from build123d import *

# Parameters (mm, degrees)
SKETCH1_R           = 10
BOSS_EXTRUDE1_DEPTH = 22
SKETCH2_R           = 3
BOSS_EXTRUDE2_DEPTH = 6


with BuildPart() as part:
    # Sketch1 → Boss-Extrude1 (new body)
    with BuildSketch(Plane.XY):
        Circle(SKETCH1_R)
    extrude(amount=BOSS_EXTRUDE1_DEPTH)

    # Sketch2 → Boss-Extrude2 (add)
    with BuildSketch(Plane.XY.offset(22)):
        Circle(SKETCH2_R)
    extrude(amount=BOSS_EXTRUDE2_DEPTH)

    # Sketch6 → Cut-Revolve3 (revolve, cut)
    with BuildSketch(Plane(origin=(0, 0, 0), x_dir=(0, 0, -1), z_dir=(1, 0, 0)), mode=Mode.PRIVATE) as cut_revolve3_sk:
        with BuildLine():
            Line((-11, 0), (-11, 10))
            Line((-11, 10), (-1, 10))
            ThreePointArc((-1, 10), (-3.928932188, 2.928932188), (-11, 0))
        make_face()
    revolve(cut_revolve3_sk.sketch.rotate(Axis((0, 0, 11), (0, 1, 0)), 180), axis=Axis((0, 0, 11), (0, 1, 0)), mode=Mode.SUBTRACT)

    # Sketch7 → Revolve1 (revolve)
    with BuildSketch(Plane(origin=(0, 0, 0), x_dir=(0, 0, -1), z_dir=(1, 0, 0)), mode=Mode.PRIVATE) as revolve1_sk:
        with BuildLine():
            Line((-4.755002002, 15), (-2.339745962, 15))
            ThreePointArc((-2.339745962, 15), (-2.339745962, 5), (-11, 0))
            Line((-11, 0), (-11, 2))
            ThreePointArc((-11, 2), (-3.788897449, 6.535898385), (-4.755002002, 15))
        make_face()
    revolve(revolve1_sk.sketch.rotate(Axis((0, 0, 11), (0, 1, 0)), 270), axis=Axis((0, 0, 11), (0, 1, 0)))


solid = part.part
Check sheet for the modelled part. Datum: model origin and axes. Units: mm. A direction names the side the tool comes from. Round coordinates to 2 decimals unless told otherwise and drop trailing zeros. Order: outer loops, then holes, each group sorted by start corner. A loop starts at its lowest first (then second) coordinate and runs counter-clockwise, first axis right, second up.
Q1. Set-up check for faces 1 (the face through (2.1, 2.4, 22)), 2 (the face through (0, 0, 0)): record each of +Z, -Z, +X, -X, +Y, -Y from which the full face is reachable in a straight line by a thin tool's end or side.
Filled sheet:
face 1: +Z
face 2: -Z, +X, -X, +Y, -Y
Q2. Cross-section at C-C, the plane z = 5.5. Enter the section's corners in (x, y).
Filled sheet:
outline: (-7.59, 6.51) arc R10 ccw (long way) to (7.59, 6.51) arc R8.35 ccw to (6.69, 15) - (2.96, 15) arc R5.81 cw (long way) to (-2.96, 15) - (-6.69, 15) arc R8.35 ccw to start
Q3. Depth check by flat-ended pin: P1, Ø5, axis at y = 10.5, z = 20.5, coming from the +X side; P2, Ø4, axis at y = 7.5, z = 8.5, coming from the -X side; P3, Ø3, axis at y = 9, z = 9.5, coming from the +X side. Enter the tip coordinate at first touch or a pass-through.
Filled sheet:
P1: stops at x = 7.13
P2: stops at x = -9.88
P3: stops at x = 10
Q4. Cross-section at B-B, the plane x = 5.75. Enter the section's corners in (y, z), plus the area to 3 significant figures.
Filled sheet:
outline: (-8.18, 0) - (8.18, 0) - (8.18, 3.02) arc R8.18 ccw to (15, 4.52) - (15, 8.56) arc R5.56 cw (long way) to (15, 13.44) - (15, 17.48) arc R8.18 ccw to (8.18, 18.98) - (8.18, 22) - (-8.18, 22) - close
area: 371 mm2
Q5. Scan lines: L1, parallel to Z at x = 6, y = 2.25; L2, parallel to Y at x = -3, z = 5; L3, parallel to X at y = 5, z = 15.5. Record each from-to range of solid material in increasing order.
Filled sheet:
L1: z = 0 to 22
L2: y = -9.54 to 5.64, 14.36 to 15
L3: x = -8.66 to -4.33, 4.33 to 8.66
Q6. Cross-section at D-D, the plane y = 6.25. Enter the section's corners in (x, z).
Filled sheet:
outline: (-7.81, 0) - (7.81, 0) - (7.81, 6) arc R9.27 ccw to (7.81, 16) - (7.81, 22) - (-7.81, 22) - (-7.81, 16) arc R9.27 ccw to (-7.81, 6) - close; hole circle Ø14.13 at (0, 11)
Q7. Cross-section at A-A, the plane y = 0. Enter the section's corners in (x, z), plus the area to 3 significant figures.
Filled sheet:
outline: (-10, 0) - (10, 0) - (10, 22) - (3, 22) - (3, 28) - (-3, 28) - (-3, 22) - (-10, 22) - close
area: 476 mm2
